Here's how the part is built. I have some questions about the finished solid (model axes, mm). Face numbers are marked on the shaded views. Coordinates: 2 decimals unless noted, no trailing zeros. Write each loop counter-clockwise with the first axis right and the second up, starting at its lowest first coordinate (ties: lowest second). Pieces come first, ordered by that corner, then holes.
Item 1: Please list where these lines run through material, in increasing order: line 1 (X direction, y = -3.35, z = 0); line 2 (X direction, y = 0, z = -0.5); line 3 (X direction, y = -0.05, z = -2).
Item 2: I want a section at D-D (x = -11.5). Please give me the cut outline in (y, z) (3 decimals).
Item 3: If we mould it in two halves opening along X, with no side actions, what happens to the marked faces 1, 2 and 3? For each: pulls with the +X half, pulls with the -X half, needs draft (parallel to the pull), parting line crosses it, or undercut.
Item 4: I want a section at C-C (x = 5). Please give me the cut outline in (y, z) (3 decimals).
Item 5: I want a section at B-B (y = -1.4). Please give me the cut outline in (x, z), and give its area (3 significant figures).
Item 6: I'm going to push flat-ended pins straight in: P1, Ø0.9, axis at x = 11.5, z = 0.5, coming from the -Y side; P2, Ø3, axis at x = -8.5, y = -3.5, coming from the -Z side; P3, Ø2, axis at y = -2.5, z = -11, coming from the -X side; P4, Ø1.5, axis at y = -1.5, z = -1.5, coming from the -X side. Where does each tip first touch, or does it pass through?
Item 7: I want a section at A-A (z = 0). Please give me the cut outline in (x, y) (3 decimals).
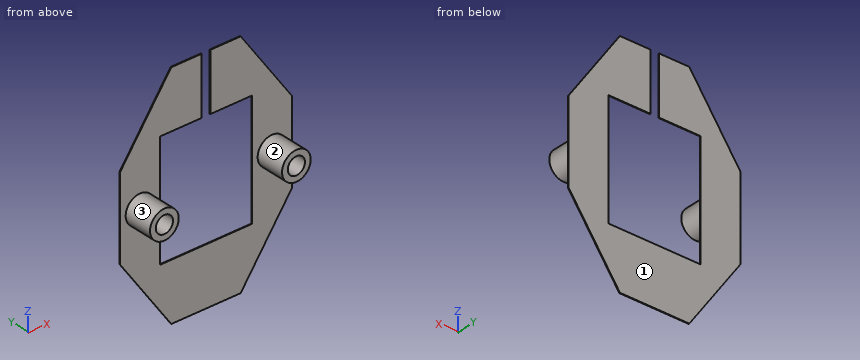
from build123d import *

# Parameters (mm, degrees)
SKETCH1_W           = 33
SKETCH1_H           = 43
BOSS_EXTRUDE1_DEPTH = 0.375
CUT_EXTRUDE1_DEPTH  = 0.25
SKETCH3_W           = 16
SKETCH3_H           = 20
CUT_EXTRUDE2_DEPTH  = 4.125
CUT_EXTRUDE3_DEPTH  = 4.125
SKETCH5_W           = 1.5
SKETCH5_H           = 10
CUT_EXTRUDE4_DEPTH  = 10
SKETCH6_W           = 11.671124307
SKETCH6_H           = 24.955330834
SKETCH6_W_2         = 23.228162705
SKETCH6_H_2         = 5.306808708
SKETCH6_W_3         = 8.676096845
SKETCH6_H_3         = 22.396436041
SKETCH6_W_4         = 27.721988928
SKETCH6_H_4         = 5.80460418
CUT_EXTRUDE5_DEPTH  = 5
SKETCH7_R           = 2.5
SKETCH7_R_2         = 1.5
BOSS_EXTRUDE2_DEPTH = 5


with BuildPart() as part:
    # Sketch1 → Boss-Extrude1 (new body)
    with BuildSketch(Plane(origin=(0, 0, 0), x_dir=(1, 0, 0), z_dir=(0, 1, 0))):
        Rectangle(SKETCH1_W, SKETCH1_H)
    extrude(amount=BOSS_EXTRUDE1_DEPTH)

    # Sketch2 → Cut-Extrude1 (cut)
    with BuildSketch(Plane.XZ):
        Polygon((5, 21.5), (16.5, 21.5), (16.5, 5), (15, 5), (15, -5), (16.5, -5), (16.5, -21.5), (5, -21.5), (5, -20), (-5, -20), (-5, -21.5), (-16.5, -21.5), (-16.5, -5), (-15, -5), (-15, 5), (-16.5, 5), (-16.5, 21.5), (-5, 21.5), (-5, 20), (5, 20), align=None)
    extrude(amount=-CUT_EXTRUDE1_DEPTH, mode=Mode.SUBTRACT)

    # Sketch3 → Cut-Extrude2 (cut)
    with BuildSketch(Plane.XZ.offset(-0.25)):
        Rectangle(SKETCH3_W, SKETCH3_H)
    extrude(amount=-CUT_EXTRUDE2_DEPTH, mode=Mode.SUBTRACT)

    # Sketch4 → Cut-Extrude3 (cut)
    with BuildSketch(Plane.XZ.offset(-0.25)):
        Polygon((-5, 21.5), (-16.5, 5), (-16.5, 21.5), align=None)
        Polygon((5, 21.5), (16.5, 5), (16.5, 21.5), align=None)
        Polygon((-16.5, -5), (-5, -21.5), (-16.5, -21.5), align=None)
        Polygon((16.5, -5), (5, -21.5), (16.5, -21.5), align=None)
    extrude(amount=-CUT_EXTRUDE3_DEPTH, mode=Mode.SUBTRACT)

    # Sketch5 → Cut-Extrude4 (cut)
    with BuildSketch(Plane.XZ.offset(-0.25)):
        with Locations((0, 15)):
            Rectangle(SKETCH5_W, SKETCH5_H)
    extrude(amount=-CUT_EXTRUDE4_DEPTH, mode=Mode.SUBTRACT)

    # Sketch6 → Cut-Extrude5 (cut, symmetric)
    with BuildSketch(Plane.XZ.offset(-0.25)):
        with Locations((20.835562154, -1.334081217)):
            Rectangle(SKETCH6_W, SKETCH6_H)
        with Locations((-0.739473345, -22.653404354)):
            Rectangle(SKETCH6_W_2, SKETCH6_H_2)
        with Locations((-19.338048423, -1.063266803)):
            Rectangle(SKETCH6_W_3, SKETCH6_H_3)
        with Locations((-0.937806624, 22.90230209)):
            Rectangle(SKETCH6_W_4, SKETCH6_H_4)
    extrude(amount=CUT_EXTRUDE5_DEPTH, both=True, mode=Mode.SUBTRACT)

    # Sketch7 → Boss-Extrude2 (add)
    # profile 1 of 2: a face of its own
    with BuildSketch(Plane(origin=(0, 0.25, 0), x_dir=(-1, 0, 0), z_dir=(0, -1, 0))):
        with Locations(Location((11.5, 0, 0), (0, 0, 270))):
            Circle(SKETCH7_R)
        with Locations(Location((11.5, 0, 0), (0, 0, 90))):
            Circle(SKETCH7_R_2, mode=Mode.SUBTRACT)
    # profile 2 of 2: a face of its own
    with BuildSketch(Plane(origin=(0, 0.25, 0), x_dir=(-1, 0, 0), z_dir=(0, -1, 0))):
        with Locations(Location((-11.5, 0, 0), (0, 0, 270))):
            Circle(SKETCH7_R)
        with Locations(Location((-11.5, 0, 0), (0, 0, 90))):
            Circle(SKETCH7_R_2, mode=Mode.SUBTRACT)
    extrude(amount=BOSS_EXTRUDE2_DEPTH)


solid = part.part
Answer:
1. line 1: x = -14 to -13, -10 to -9, 9 to 10, 13 to 14
1. line 2: x = -13.95 to -12.91, -10.09 to -9.05, 9.05 to 10.09, 12.91 to 13.95
1. line 3: x = -13 to -10, 10 to 13
2. outline: (-4.75, -2.5) - (0.25, -2.5) - (0.25, -12.174) - (0.375, -12.174) - (0.375, 12.174) - (0.25, 12.174) - (0.25, 2.5) - (-4.75, 2.5) - (-4.75, 1.5) - (0.25, 1.5) - (0.25, -1.5) - (-4.75, -1.5) - close
3. face 1: needs draft
3. face 2: undercut
3. face 3: undercut
4. outline: (0.25, -20) - (0.375, -20) - (0.375, -10) - (0.25, -10) - close; (0.25, 10) - (0.375, 10) - (0.375, 20) - (0.25, 20) - close
5. outline: circle Ø5 at (-11.5, 0); circle Ø5 at (11.5, 0); hole circle Ø3 at (-11.5, 0); hole circle Ø3 at (11.5, 0)
5. area: 25.1 mm2
6. P1: stops at y = 0.25
6. P2: stops at z = -2
6. P3: passes through
6. P4: stops at x = -13.88
7. outline: (-15, 0.25) - (-14, 0.25) - (-14, -4.75) - (-13, -4.75) - (-13, 0.25) - (-10, 0.25) - (-10, -4.75) - (-9, -4.75) - (-9, 0.25) - (-8, 0.25) - (-8, 0.375) - (-15, 0.375) - close; (8, 0.25) - (9, 0.25) - (9, -4.75) - (10, -4.75) - (10, 0.25) - (13, 0.25) - (13, -4.75) - (14, -4.75) - (14, 0.25) - (15, 0.25) - (15, 0.375) - (8, 0.375) - close
